```python
from build123d import *

# Parameters (mm, degrees)
BOSS_EXTRUDE1_DEPTH = 2
SKETCH2_R           = 1
CUT_EXTRUDE1_DEPTH  = 10


with BuildPart() as part:
    # Sketch1 → Boss-Extrude1 (new body)
    with BuildSketch(Plane.XY):
        with BuildLine():
            ThreePointArc((-75.246672681, -2.507158848), (-74.879445737, -2.042044212), (-74.313447388, -1.866450586))
            Line((-74.313447388, -1.866450586), (74.313447388, -1.866450586))
            ThreePointArc((74.313447388, -1.866450586), (74.955034485, -2.065494638), (75.371304372, -2.592725061))
            Line((75.371304372, -2.592725061), (94.116450586, -51.281416525))
            Line((94.116450586, -51.281416525), (-94.294779137, -51.982760032))
            Line((-94.294779137, -51.982760032), (-75.246672681, -2.507158848))
        make_face()
        with BuildLine():
            Line((-94.294779137, -51.982760032), (-75.246672681, -2.507158848))
            ThreePointArc((-75.246672681, -2.507158848), (-74.879445737, -2.042044212), (-74.313447388, -1.866450586))
            Line((-74.313447388, -1.866450586), (74.313447388, -1.866450586))
            ThreePointArc((74.313447388, -1.866450586), (74.955034485, -2.065494638), (75.371304372, -2.592725061))
            Line((75.371304372, -2.592725061), (94.116450586, -51.281416525))
            Line((94.116450586, -51.281416525), (96.116450586, -51.281416525))
            Line((96.116450586, -51.281416525), (77.113123267, -1.922124787))
            ThreePointArc((77.113123267, -1.922124787), (76.011442435, -0.526780879), (74.313447388, 0))
            Line((74.313447388, 0), (25, 0))
            Line((25, 0), (-25, 0))
            Line((-25, 0), (-74.313447388, 0))
            ThreePointArc((-74.313447388, 0), (-76.011442435, -0.526780879), (-77.113123267, -1.922124787))
            Line((-77.113123267, -1.922124787), (-96.116450586, -51.281416525))
            Line((-96.116450586, -51.281416525), (-94.294779137, -51.982760032))
        make_face()
    extrude(amount=BOSS_EXTRUDE1_DEPTH)

    # Sketch2 → Cut-Extrude1 (cut)
    with BuildSketch(Plane.XY.offset(2)):
        with Locations((0, -12)):
            Circle(SKETCH2_R)
    extrude(amount=-CUT_EXTRUDE1_DEPTH, mode=Mode.SUBTRACT)


solid = part.part
```
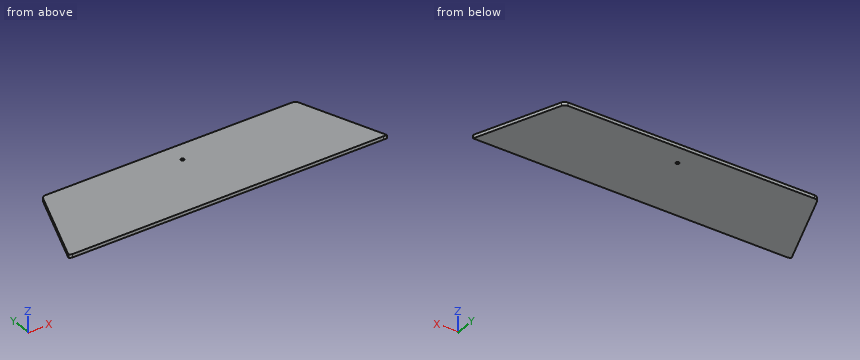
The model under review builds one solid part; all positions refer to its coordinate system, in mm. Round coordinates to 2 decimals unless told otherwise and drop trailing zeros. Loops run counter-clockwise (first coordinate to the right, second up) from the corner with the lowest first, then second, coordinate; pieces in that order, holes last. Notation, with made-up numbers: (-11.75, -38) -> (6.25, -38) arc R11 ccw to (6.25, -34) -> close; hole circle Ø8 at (44.5, 16.5). An arc over 180 degrees is marked (long way). Answer as a JSON object with one key per item and string values. Group by question number.
1) For pin 1 Ø0.6 at (x, z) = (94.5, 1.5) entering from -Y; pin 2 Ø1.6 at (x, y) = (0, -12) entering from +Z, all flat-tipped, find the tip position at first contact; note any pin that passes through.
2) We need section B-B on y = -22. Write out the cut boundary in (x, z), then the cut area to 3 significant figures.
3) We need section A-A on z = 0.8. Write out the cut boundary in (x, y).
4) For line 1 (Y direction, x = 0, z = 0.9); line 2 (Y direction, x = 5.5, z = 1.2); line 3 (X direction, y = -48, z = 0.75), list the stretches that pass through material, from the lowest coordinate up. Write a range as [from, to].
Result set:
{
 "1": {"pin 1": "y = -51.28", "pin 2": "through"},
 "2": {"outline": "(-84.84, 0) -> (84.84, 0) -> (84.84, 2) -> (-84.84, 2) -> close", "area": "339 mm²"},
 "3": {"outline": "(-96.12, -51.28) -> (-94.29, -51.98) -> (94.12, -51.28) -> (96.12, -51.28) -> (77.11, -1.92) arc R3 ccw to (74.31, 0) -> (-74.31, 0) arc R3 ccw to (-77.11, -1.92) -> close; hole circle Ø2 at (0, -12)"},
 "4": {"line 1": "[-51.63, -13], [-11, 0]", "line 2": "[-51.61, 0]", "line 3": "[-94.85, 94.85]"}
}
